```python
from build123d import *

# Parameters (mm, degrees)
BOSS_EXTRUDE1_DEPTH = 1.5
SKETCH2_W           = 6
SKETCH2_H           = 6.35
BOSS_EXTRUDE2_DEPTH = 3


with BuildPart() as part:
    # Sketch1 → Boss-Extrude1 (new, symmetric)
    with BuildSketch(Plane(origin=(0, 0, 0), x_dir=(1, 0, 0), z_dir=(0, 1, 0))):
        with BuildLine():
            Line((14.2875, -4.7625), (-14.2875, -4.7625))
            ThreePointArc((-14.2875, -4.7625), (-15.410032015, -4.297532015), (-15.875, -3.175))
            Line((-15.875, -3.175), (-15.875, 3.175))
            ThreePointArc((-15.875, 3.175), (-15.410032015, 4.297532015), (-14.2875, 4.7625))
            Line((-14.2875, 4.7625), (14.2875, 4.7625))
            ThreePointArc((14.2875, 4.7625), (15.410032015, 4.297532015), (15.875, 3.175))
            Line((15.875, 3.175), (15.875, -3.175))
            ThreePointArc((15.875, -3.175), (15.410032015, -4.297532015), (14.2875, -4.7625))
        make_face()
    extrude(amount=BOSS_EXTRUDE1_DEPTH, both=True)

    # Sketch2 → Boss-Extrude2 (add)
    with BuildSketch(Plane(origin=(0, 1.5, 0), x_dir=(1, 0, 0), z_dir=(0, 1, 0))):
        with Locations((-18.875, 0)):
            Rectangle(SKETCH2_W, SKETCH2_H)
    boss_extrude2 = extrude(amount=-BOSS_EXTRUDE2_DEPTH)

    # Mirror1: Boss-Extrude2 across plane
    add(boss_extrude2.mirror(Plane(origin=(0, 0, 0), x_dir=(0, 0, 1), z_dir=(1, 0, 0))))


solid = part.part
```
Geometry check sheet. Reference: the model listing, model coordinates, mm. A direction names the side the tool comes from. Give positions to 0.01 mm unless a question says otherwise; leave off trailing zeros. Order: outer loops, then holes, each group sorted by start corner. A loop starts at its lowest first (then second) coordinate and runs counter-clockwise, first axis right, second up. Notation, with made-up numbers: (88, 2.25) - (142, 2.25) arc R18 cw to (142, 34.25) - close; hole circle Ø3 at (-23.75, 13.25). An arc over 180 degrees is marked (long way). Answer in a Markdown table with one row per item. Add a question column.
Q1. Gauge pin test, flat ends, axial feed: pin 1 (0.9 mm diameter, centred on x = 18, y = 0, fed in from -Z) (3 decimals); pin 2 (1.5 mm diameter, centred on x = 18, y = 0.5, fed in from +Z) (3 decimals). Record the tip position at first contact, or that the pin passes through.
Q2. Cross-section at A-A, the plane z = 4. Enter the section's corners in (x, y), then the cut area to 3 significant figures.
Q3. Material ranges on probe 1 along Z at (x, y) = (19, -0.4) (3 decimals); probe 2 along Z at (x, y) = (-15, -0.75); probe 3 along X at (y, z) = (0.7, 4), recorded low to high. Write a range as from..to.
Q4. Tool access check on faces 1 (the flat face through (-19, 0, 3.175)), 2 (the flat face through (19, 0, 3.175)), 3 (the flat face through (19, 0, -3.175)). Record the directions out of +Z, -Z, +X, -X, +Y, -Y that give a thin tool (end or side, any length) a straight path to the whole face; none if there is none.
Check values:
| question | item | result |
|---|---|---|
| 1 | pin 1 | stops at z = -3.175 |
| 1 | pin 2 | stops at z = 3.175 |
| 2 | outline | (-15.64, -1.5) - (15.64, -1.5) - (15.64, 1.5) - (-15.64, 1.5) - close |
| 2 | area | 93.9 mm^2 |
| 3 | probe 1 | z = -3.175..3.175 |
| 3 | probe 2 | z = -4.59..4.59 |
| 3 | probe 3 | x = -15.64..15.64 |
| 4 | face 1 | +Z, -X, +Y, -Y |
| 4 | face 2 | +Z, +X, +Y, -Y |
| 4 | face 3 | -Z, +X, +Y, -Y |
